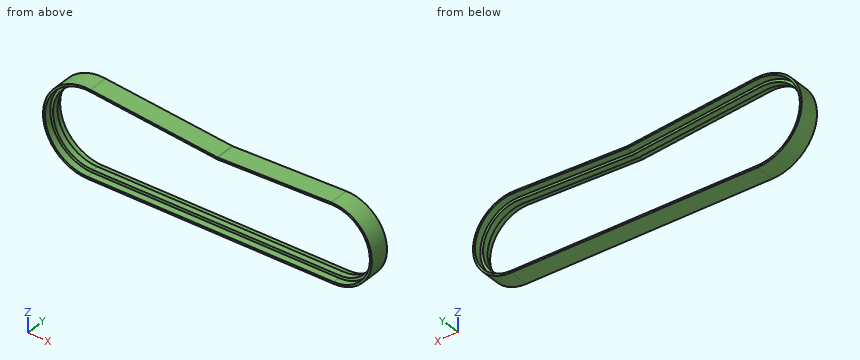
```python
from build123d import *

# Parameters (mm, degrees)
BOSS_EXTRUDE1_DEPTH = 5
BOSS_EXTRUDE2_DEPTH = 1.5


with BuildPart() as part:
    # Sketch1 → Boss-Extrude1 (new, symmetric)
    with BuildSketch(Plane(origin=(0, 0, 0), x_dir=(1, 0, 0), z_dir=(0, 1, 0))):
        with BuildLine():
            Line((0.434583333, 22.345774485), (126.386944444, 19.896237684))
            ThreePointArc((126.386944444, 19.896237684), (145.888566517, -0.674478997), (125.038127363, -19.876740201))
            Line((125.038127363, -19.876740201), (67.116731829, -16.970417062))
            ThreePointArc((67.116731829, -16.970417062), (66.886386328, -16.966450661), (66.65627889, -16.977646615))
            Line((66.65627889, -16.977646615), (1.820273578, -22.275751482))
            ThreePointArc((1.820273578, -22.275751482), (-22.339230959, -0.693729175), (0.434583333, 22.345774485))
        make_face()
        with BuildLine():
            Line((0.415138889, 21.345963546), (126.3675, 18.896426746))
            ThreePointArc((126.3675, 18.896426746), (144.88856319, -0.657404457), (125.052845875, -18.876252252))
            Line((125.052845875, -18.876252252), (67.150013324, -15.970860547))
            ThreePointArc((67.150013324, -15.970860547), (66.862262413, -15.966714067), (66.574834882, -15.980968697))
            Line((66.574834882, -15.980968697), (1.73882957, -21.279073564))
            ThreePointArc((1.73882957, -21.279073564), (-21.339712795, -0.662689838), (0.415138889, 21.345963546))
        make_face(mode=Mode.SUBTRACT)
    extrude(amount=BOSS_EXTRUDE1_DEPTH, both=True)

    # Sketch8 → Boss-Extrude2 (add, symmetric)
    with BuildSketch(Plane(origin=(0, 0, 0), x_dir=(1, 0, 0), z_dir=(0, 1, 0))):
        with BuildLine():
            Line((67.1403688, -16.170628229), (125.04282308, -19.076000953))
            ThreePointArc((125.04282308, -19.076000953), (145.088442165, -0.664361118), (126.371388889, 19.096388933))
            Line((126.371388889, 19.096388933), (0.419027778, 21.545925734))
            ThreePointArc((0.419027778, 21.545925734), (-21.539616428, -0.668897706), (1.755118371, -21.478409147))
            Line((1.755118371, -21.478409147), (66.591123683, -16.18030428))
            ThreePointArc((66.591123683, -16.18030428), (66.865591568, -16.166686447), (67.1403688, -16.170628229))
        make_face()
        with BuildLine():
            Line((67.217731767, -14.572497151), (125.12300544, -17.478011344))
            ThreePointArc((125.12300544, -17.478011344), (143.489410361, -0.60870783), (126.340277778, 17.496691431))
            Line((126.340277778, 17.496691431), (0.387916667, 19.946228231))
            ThreePointArc((0.387916667, 19.946228231), (-19.940387366, -0.619234767), (1.624807959, -19.883724478))
            Line((1.624807959, -19.883724478), (66.460813271, -14.58561961))
            ThreePointArc((66.460813271, -14.58561961), (66.839061833, -14.566905785), (67.217731767, -14.572497151))
        make_face(mode=Mode.SUBTRACT)
    extrude(amount=BOSS_EXTRUDE2_DEPTH, both=True)


solid = part.part
```
Can you work these out from the model? Positions are in its coordinate system, mm. Round coordinates to 2 decimals unless told otherwise and drop trailing zeros. Loops run counter-clockwise (first coordinate to the right, second up) from the corner with the lowest first, then second, coordinate; pieces in that order, holes last. Notation, with made-up numbers: M 28.25,48.25 L 46.25,48.25 A14 cw 46.25,64.25 Z; hole C 5,-2.75 d3. An arc over 180 degrees is marked long. Write item = value, one per line. Start each with the question number.
(1) Suppose I cut it at C-C on x = 107.5. Write out the boundary of the cut face in (y, z).
(2) Suppose I cut it at A-A on z = 0. Write out the boundary of the cut face in (x, y), plus the area to 3 significant figures.
(3) I'm going to push flat-ended pins straight in: P1, Ø4, axis at x = 125.5, y = 0.5, coming from the +Z side; P2, Ø13, axis at x = 32.5, z = 9, coming from the -Y side; P3, Ø1.5, axis at y = -4, z = 17.5, coming from the -X side; P4, Ø6, axis at y = -1, z = 16.5, coming from the -X side. Where does each tip first touch, or does it pass through?
(4) I need wall thicknesses on line 1 along X through (y, z) = (-4, 0); line 2 along Z through (x, y) = (123, -2.25); line 3 along X through (y, z) = (2, -2.5). Which ranges of each line are inside material? Lowest first, please.
(5) Suppose I cut it at B-B on y = 3. Write out the boundary of the cut face in (x, z), plus the area to 3 significant figures.
Answer block:
q1.outline = M -5,-20.26 L 5,-20.26 L 5,-19.26 L 1.5,-19.26 L 1.5,-17.86 L -1.5,-17.86 L -1.5,-19.26 L -5,-19.26 Z; M -5,18 L -1.5,18 L -1.5,16.59 L 1.5,16.59 L 1.5,18 L 5,18 L 5,19 L -5,19 Z
q2.outline = M -22.35,-5 L -21.35,-5 L -21.35,-1.5 L -19.95,-1.5 L -19.95,1.5 L -21.35,1.5 L -21.35,5 L -22.35,5 Z; M 143.5,-1.5 L 144.9,-1.5 L 144.9,-5 L 145.9,-5 L 145.9,5 L 144.9,5 L 144.9,1.5 L 143.5,1.5 Z
q2.area = 28.4 mm²
q3.P1 = 19.9
q3.P2 = through
q3.P3 = -14.8
q3.P4 = -17.81
q4.line_1 = -22.35 to -21.35, 144.9 to 145.9
q4.line_2 = -19.96 to -18.96, 18.77 to 19.77
q4.line_3 = -22.21 to -21.2, 144.73 to 145.74
q5.outline = M 0.43,-22.35 L 126.39,-19.9 A19.9 ccw long 125.04,19.88 L 67.12,16.97 A3.5 cw 66.66,16.98 L 1.82,22.28 A22.35 ccw long Z; hole M 0.42,-21.35 L 126.37,-18.9 A18.9 ccw long 125.05,18.88 L 67.15,15.97 A4.5 cw 66.57,15.98 L 1.74,21.28 A21.35 ccw long Z
q5.area = 382 mm²
